```python
from build123d import *

# Parameters (mm, degrees)
F0_R     = 8
F2_DEPTH = 10
F3_DEPTH = 45
F5_DEPTH = 10


with BuildPart() as f2:
    # F0 (on Front) → F2 (new body)
    with BuildSketch(Plane.XZ):
        with BuildLine():
            Line((-14.09482, 44.536495), (-71.326971, -54.5925))
            Line((-71.326971, -54.5925), (73.482672, -54.5925))
            Line((73.482672, -54.5925), (16.25052, 44.536495))
            ThreePointArc((16.25052, 44.536495), (1.07785, 53.29644), (-14.09482, 44.536495))
        make_face()
        with Locations((1.07785, 35.77655)):
            Circle(F0_R, mode=Mode.SUBTRACT)
    extrude(amount=F2_DEPTH)

    # F1 (on Front) → F3 (join)
    with BuildSketch(Plane.XZ):
        Polygon((73.503241, -54.489337), (-71.249463, -54.489337), (-71.249463, -61.854444), (-71.249463, -65.678634), (73.503241, -65.678634), (73.503241, -61.854444), align=None)
    extrude(amount=F3_DEPTH)

    # F4 (on face) → F5 (join)
    with BuildSketch(Plane.XZ.offset(45)):
        Polygon((-71.249463, -54.64355), (-71.249463, -65.678634), (-31.249463, -65.678634), (-31.249463, -38.922109), (-51.249463, -38.922109), align=None)
        Polygon((33.34011, -65.918161), (73.34011, -65.918161), (73.34011, -54.64355), (53.34011, -37.731093), (33.34011, -37.731093), align=None)
    extrude(amount=F5_DEPTH)


solid = f2.part
```
Could you check a few things on this model? Use its own coordinates, in mm. A direction names the side the tool comes from. Round coordinates to 2 decimals unless told otherwise and drop trailing zeros. Loops run counter-clockwise (first coordinate to the right, second up) from the corner with the lowest first, then second, coordinate; pieces in that order, holes last. Notation, with made-up numbers: (38.5, -31) -> (43.5, -31) arc R21 ccw to (43.5, -4) -> close; hole circle Ø8 at (10.5, 74.5). An arc over 180 degrees is marked (long way). Put each result on its own line as item: value.
Q1. For pin 1 Ø9 at (x, z) = (12.5, -62.5) entering from -Y; pin 2 Ø1 at (x, z) = (-16, -50) entering from -Y; pin 3 Ø11 at (x, y) = (-42, -51) entering from +Z; pin 4 Ø11 at (y, z) = (-49.5, -60) entering from +X, each with a flat end and sliding along its axis, tell me the tip position at first contact or that it passes through.
Checks:
pin 1: y = -45
pin 2: y = -10
pin 3: z = -38.92
pin 4: x = 73.5
Q2. Please list where these lines run through material, in increasing order: line 1 (Z direction, x = 8, y = -37.5); line 2 (Y direction, x = 31, z = -2); line 3 (X direction, y = -4, z = 43). Write a range as from..to.
Checks:
line 1: -65.68..-54.49
line 2: -10..0
line 3: -14.98..-2.36, 4.52..17.14
Q3. Thinking about a two-plate mould opening in X: for faces 1 (the cylindrical face through (-0.656, -4.93, 27.967)), 2 (the flat face through (-71.249, -27, -60)), 3 (the flat face through (1, -45, -60)), 4 (the flat face through (43, -50, -37.731)), which applies, pulls with the +X half, pulls with the -X half, needs draft (parallel to the pull), parting line crosses it, or undercut?
Checks:
face 1: undercut
face 2: pulls with the -X half
face 3: undercut
face 4: needs draft
Q4. I want a section at C-C on x = -44. Write out the boundary of the cut face in (y, z), and give its area (3 significant figures).
Checks:
outline: (-55, -65.68) -> (0, -65.68) -> (0, -7.26) -> (-10, -7.26) -> (-10, -54.49) -> (-45, -54.49) -> (-45, -38.92) -> (-55, -38.92) -> close
area: 1,240 mm2
Q5. Which directions (+Z, -Z, +X, -X, +Y, -Y) give clear straight access to the entire face, cutting with the end or side of a thin tool? Please do faces 5 (the flat face through (-41, -50, -38.922)), 6 (the flat face through (49, -45, -46)), 7 (the cylindrical face through (1.335, -4.93, 53.295)), 8 (the flat face through (63.48, -49.93, -46.306)), 9 (the flat face through (-47, -55, -52)).
Checks:
face 5: +Z, -X, -Y
face 6: +Z, +X, -X
face 7: +Z, +Y, -Y
face 8: +Z, +X, -Y
face 9: +Z, -Z, +X, -X, -Y
Q6. I want a section at B-B on z = 39.5. Write out the boundary of the cut face in (x, y), and give its area (3 significant figures).
Checks:
outline: (-17, -10) -> (-6, -10) -> (-6, 0) -> (-17, 0) -> close; (8.16, -10) -> (19.16, -10) -> (19.16, 0) -> (8.16, 0) -> close
area: 220 mm2
Q7. I want a section at D-D on z = 10.5. Write out the boundary of the cut face in (x, y).
Checks:
outline: (-33.75, -10) -> (35.9, -10) -> (35.9, 0) -> (-33.75, 0) -> close
Q8. I want a section at A-A on y = -47. Write out the boundary of the cut face in (x, z).
Checks:
outline: (-71.25, -65.68) -> (-31.25, -65.68) -> (-31.25, -38.92) -> (-51.25, -38.92) -> (-71.25, -54.64) -> close; (33.34, -65.92) -> (73.34, -65.92) -> (73.34, -54.64) -> (53.34, -37.73) -> (33.34, -37.73) -> close
